Design review of the part built by this model. Coordinates are the model's own, in mm. Face numbers are marked on the shaded views. A direction names the side the tool comes from. Give positions to 0.01 mm unless a question says otherwise; leave off trailing zeros. Loops run counter-clockwise (first coordinate to the right, second up) from the corner with the lowest first, then second, coordinate; pieces in that order, holes last.
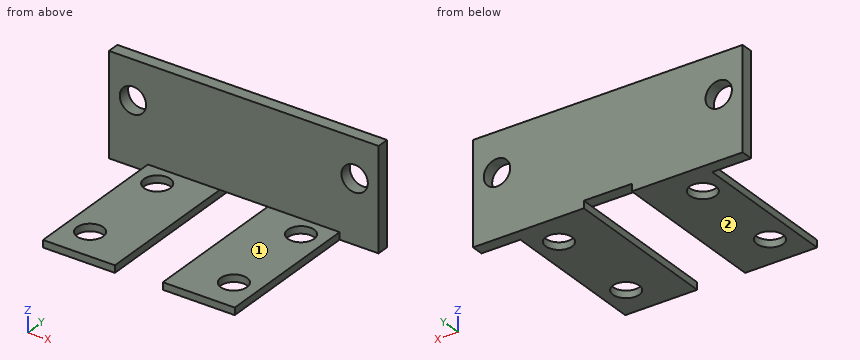
from build123d import *

# Parameters (mm, degrees)
F0_W      = 45
F0_H      = 27
F1_DEPTH  = 17
F2_W      = 25
F2_H      = 15.8
F3_DEPTH  = 45.001
F4_W      = 8
F4_H      = 27
F5_DEPTH  = 1.201
F7_D      = 4.4
F9_D      = 4.4
F10_W     = 6.5
F10_H     = 25
F11_DEPTH = 1.201


with BuildPart() as f1:
    # F0 (on Top) → F1 (new body)
    with BuildSketch(Plane.XY):
        Rectangle(F0_W, F0_H)
    extrude(amount=F1_DEPTH)

    # F2 (on face) → F3 (cut, through all)
    with BuildSketch(Plane.YZ.offset(22.5)):
        with Locations((-1, 9.1)):
            Rectangle(F2_W, F2_H)
    extrude(amount=-F3_DEPTH, mode=Mode.SUBTRACT)

    # F4 (on face) → F5 (cut, through all)
    with BuildSketch(Plane.XY.offset(1.2)):
        Rectangle(F4_W, F4_H)
    extrude(amount=-F5_DEPTH, mode=Mode.SUBTRACT)

    # F7 (through all)
    with Locations(Plane(origin=(0, 0, 0), x_dir=(1, 0, 0), z_dir=(0, 0, -1))):
        with Locations((-12, 8), (12, 8), (12, -8), (-12, -8)):
            Hole(F7_D / 2)

    # F9 (through all)
    with Locations(Plane(origin=(0, 13.5, 0), x_dir=(-1, 0, 0), z_dir=(0, 1, 0))):
        with Locations((18.5, 10.5), (-18.5, 10.5)):
            Hole(F9_D / 2)

    # F10 (on face) → F11 (cut, through all)
    with BuildSketch(Plane.XY.offset(1.2)):
        with Locations((-19.25, -1)):
            Rectangle(F10_W, F10_H)
        with Locations((19.25, -1)):
            Rectangle(F10_W, F10_H)
    extrude(amount=-F11_DEPTH, mode=Mode.SUBTRACT)


solid = f1.part
Q1. Take a section at B-B (y = -11). Give the boundary of the cut face in (x, z).
Results:
outline: (-16, 0) - (-4, 0) - (-4, 1.2) - (-16, 1.2) - close; (4, 0) - (16, 0) - (16, 1.2) - (4, 1.2) - close
Q2. Take a section at A-A (x = -18.5). Give the boundary of the cut face in (y, z), plus the area to 3 significant figures.
Results:
outline: (11.5, 0) - (13.5, 0) - (13.5, 8.3) - (11.5, 8.3) - close; (11.5, 12.7) - (13.5, 12.7) - (13.5, 17) - (11.5, 17) - close
area: 25.2 mm2
Q3. Wall thickness on line 1 (Y direction, x = 12, z = 0.2); line 2 (X direction, y = 8, z = 0.55); line 3 (X direction, y = -7.5, z = 1): over which ranges is each line inside the solid? List them lowest first.
Results:
line 1: y = -13.5 to -10.2, -5.8 to 5.8, 10.2 to 13.5
line 2: x = -16 to -14.2, -9.8 to -4, 4 to 9.8, 14.2 to 16
line 3: x = -16 to -14.14, -9.86 to -4, 4 to 9.86, 14.14 to 16
Q4. Take a section at C-C (x = -12). Give the boundary of the cut face in (y, z).
Results:
outline: (-13.5, 0) - (-10.2, 0) - (-10.2, 1.2) - (-13.5, 1.2) - close; (-5.8, 0) - (5.8, 0) - (5.8, 1.2) - (-5.8, 1.2) - close; (10.2, 0) - (13.5, 0) - (13.5, 17) - (11.5, 17) - (11.5, 1.2) - (10.2, 1.2) - close
Q5. Take a section at D-D (y = -8). Give the boundary of the cut face in (x, z).
Results:
outline: (-16, 0) - (-14.2, 0) - (-14.2, 1.2) - (-16, 1.2) - close; (-9.8, 0) - (-4, 0) - (-4, 1.2) - (-9.8, 1.2) - close; (4, 0) - (9.8, 0) - (9.8, 1.2) - (4, 1.2) - close; (14.2, 0) - (16, 0) - (16, 1.2) - (14.2, 1.2) - close
Q6. Tool access review of the marked faces 1 and 2: name each direction out of +Z, -Z, +X, -X, +Y, -Y from which nothing blocks a thin tool from reaching the whole face with its end or side.
Results:
face 1: +Z, +X, -X, -Y
face 2: -Z, +X, -X, +Y, -Y
Q7. Insertion check: pin 1 (3.5 mm diameter, centred on x = 9.5, y = 5, fed in from +Z); pin 2 (8 mm diameter, centred on y = 4, z = 9.5, fed in from +X); pin 3 (10 mm diameter, centred on x = 11, z = 10.5, fed in from -Y); pin 4 (1 mm diameter, centred on y = -7, z = 0.5, fed in from +X). Each pin has a flat end and moves straight along its axis. Give the tip position at first contact, or say it passes through.
Results:
pin 1: stops at z = 1.2
pin 2: passes through
pin 3: stops at y = 11.5
pin 4: stops at x = 16
